from build123d import *

# Parameters (mm, degrees)
SCHIZZO1_W               = 25
SCHIZZO1_H               = 21.5
ESTRUSIONE1_DEPTH        = 115
SCHIZZO6_W               = 103
SCHIZZO6_H               = 23.639461627
TAGLIO_ESTRUSIONE4_DEPTH = 84
SCHIZZO7_R               = 5.5
ESTRUSIONE4_DEPTH        = 103
SMUSSO1_SIZE             = 0.803847577
SMUSSO1_SIZE_2           = 3
SCHIZZO8_R               = 3
TAGLIO_ESTRUSIONE5_DEPTH = 8.5


with BuildPart() as part:
    # Schizzo1 → Estrusione1 (new body)
    with BuildSketch(Plane.XY):
        with Locations((12.5, 10.75)):
            Rectangle(SCHIZZO1_W, SCHIZZO1_H)
    extrude(amount=ESTRUSIONE1_DEPTH)

    # Schizzo6 → Taglio-Estrusione4 (cut)
    with BuildSketch(Plane(origin=(25, 0, 0), x_dir=(0, 0, -1), z_dir=(1, 0, 0))):
        with Locations((-57.5, 20.319730814)):
            Rectangle(SCHIZZO6_W, SCHIZZO6_H)
    extrude(amount=-TAGLIO_ESTRUSIONE4_DEPTH, mode=Mode.SUBTRACT)

    # Schizzo7 → Estrusione4 (add)
    with BuildSketch(Plane.XY.offset(6)):
        with Locations(Location((6, 17, 0), (0, 0, 125.096801228))):
            Circle(SCHIZZO7_R)
        with Locations(Location((18.5, 17, 0), (0, 0, 125.096801228))):
            Circle(SCHIZZO7_R)
    extrude(amount=ESTRUSIONE4_DEPTH)

    # Smusso1
    # the kernel refuses this chamfer: 3, 0.803847577 mm, written as the material it takes off along each edge
    with BuildSketch(Plane(origin=(0, 21.5, -7.790164711), x_dir=(-0.13751244702128895, -0.9905000388259545, 0), z_dir=(0, 0, 1)), Plane(origin=(0, 21.5, 109), x_dir=(-0.13751244702128895, -0.9905000388259545, 0), z_dir=(0, 0, 1))) as smusso1_piece_1:
        Polygon((SMUSSO1_SIZE * 0.990500039187, SMUSSO1_SIZE * 0.137512447071), (-SMUSSO1_SIZE_2 * 0.137512447021, SMUSSO1_SIZE_2 * 0.990500038826), (0, 0), align=None)
    extrude(amount=13.790164711, mode=Mode.SUBTRACT)
    with BuildSketch(Plane(origin=(25, 21.5, -7.790164711), x_dir=(0.13751244702128734, -0.9905000388259546, 0), z_dir=(0, 0, 1)), Plane(origin=(25, 21.5, 101.209835289), x_dir=(0.13751244702128734, -0.9905000388259546, 0), z_dir=(0, 0, 1))) as smusso1_piece_2:
        Polygon((SMUSSO1_SIZE * 0.990500039187, -SMUSSO1_SIZE * 0.137512447071), (-SMUSSO1_SIZE_2 * 0.137512447021, -SMUSSO1_SIZE_2 * 0.990500038826), (0, 0), align=None)
    extrude(amount=21.580329421, mode=Mode.SUBTRACT)

    # Schizzo8 → Taglio-Estrusione5 (cut)
    with BuildSketch(Plane.XZ):
        with Locations(Location((12, 105.5, 0), (0, 0, 270))):
            Circle(SCHIZZO8_R)
        with Locations(Location((12, 9.5, 0), (0, 0, 270))):
            Circle(SCHIZZO8_R)
    extrude(amount=-TAGLIO_ESTRUSIONE5_DEPTH, mode=Mode.SUBTRACT)


solid = part.part
The model under review builds one solid part; all positions refer to its coordinate system, in mm. A direction names the side the tool comes from. Round coordinates to 2 decimals unless told otherwise and drop trailing zeros. Loops run counter-clockwise (first coordinate to the right, second up) from the corner with the lowest first, then second, coordinate; pieces in that order, holes last. Notation, with made-up numbers: (66.5, 78.25) - (88.5, 78.25) arc R13 cw to (88.5, 101.25) - close; hole circle Ø3 at (-24, 32.5). An arc over 180 degrees is marked (long way). Use CSV: the item, a comma, the result in double quotes.
(1) For line 1 (X direction, y = 5, z = 105.5); line 2 (Y direction, x = 5.75, z = 49); line 3 (Z direction, x = 10.75, y = 13), list the stretches that pass through material, from the lowest coordinate up.
Working result:
line 1,"x = 0 to 9, 15 to 25"
line 2,"y = 0 to 8.5, 11.51 to 22.49"
line 3,"z = 0 to 6, 109 to 115"
(2) Take a section at B-B, the plane x = 6. Give the boundary of the cut face in (y, z), plus the area to 3 significant figures.
Working result:
outline,"(0, 0) - (21.5, 0) - (21.5, 6) - (22.5, 6) - (22.5, 109) - (21.5, 109) - (21.5, 115) - (0, 115) - close; hole (8.5, 6) - (11.5, 6) - (11.5, 109) - (8.5, 109) - close"
area,"2,270 mm^2"
(3) Clearance check with flat-ended pins moving along their axes: P1, Ø1.5, axis at y = 15.5, z = 20.5, coming from the +X side; P2, Ø3, axis at x = 13.5, z = 113, coming from the +Y side; P3, Ø3.5, axis at x = 12, z = 9.5, coming from the +Y side. State where each tip first meets the part, or that it passes through.
Working result:
P1,"stops at x = 23.95"
P2,"stops at y = 21.5"
P3,"stops at y = 20.49"
(4) The part is to be moulded in two halves that separate along Y. For faces 1 (the flat face through (12, 0, 57)), 2 (the flat face through (12, 11, 0)), 3 (the flat face through (23.5, 21.1, 3)), 4 (the cylindrical face through (1.95, 13.28, 56.78)), say which applies: pulls with the +Y half, pulls with the -Y half, needs draft (parallel to the pull), parting line crosses it, or undercut.
Working result:
face 1,"pulls with the -Y half"
face 2,"needs draft"
face 3,"pulls with the +Y half"
face 4,"undercut"
(5) Machinability: for faces 5 (the flat face through (12, 21.5, 3)), 6 (the flat face through (12, 21.5, 112)), 7 (the cylindrical face through (10.2, 4.2, 107.9)), 8 (the cylindrical face through (14.45, 13.28, 56.78)), which of the approach directions +Z, -Z, +X, -X, +Y, -Y give a long, thin tool a straight path to every point of the face, cutting with its end or side? Answer none if there is none.
Working result:
face 5,"-Z, +X, -X, +Y"
face 6,"+Z, +X, -X, +Y"
face 7,"-Y"
face 8,"none"
(6) Take a section at A-A, the plane y = 17. Give the boundary of the cut face in (x, z), plus the area to 3 significant figures.
Working result:
outline,"(0, 0) - (25, 0) - (25, 6) - (24, 6) - (24, 109) - (25, 109) - (25, 115) - (0, 115) - (0, 109) - (0.5, 109) - (0.5, 6) - (0, 6) - close; hole (11.5, 6) - (13, 6) - (13, 109) - (11.5, 109) - close"
area,"2,570 mm^2"
(7) Take a section at C-C, the plane z = 105.5. Give the boundary of the cut face in (x, y).
Working result:
outline,"(0, 0) - (9, 0) - (9, 8.5) - (0, 8.5) - close; circle Ø11 at (6, 17); circle Ø11 at (18.5, 17); (15, 0) - (25, 0) - (25, 8.5) - (15, 8.5) - close"
(8) Take a section at D-D, the plane y = 2. Give the boundary of the cut face in (x, z), plus the area to 3 significant figures.
Working result:
outline,"(0, 0) - (25, 0) - (25, 115) - (0, 115) - close; hole circle Ø6 at (12, 9.5); hole circle Ø6 at (12, 105.5)"
area,"2,820 mm^2"
